from build123d import *

# Parameters (mm, degrees)
CROQUIS1_W            = 42.3
CROQUIS1_H            = 42.3
EXTRUDE_FEATURE_DEPTH = 7.6
SKETCH2_R             = 29.910616844
SKETCH2_R_2           = 27
CUT_EXTRUDE1_DEPTH    = 8.6
CROQUIS5_R            = 1.5
CORTAR_EXTRUIR2_DEPTH = 22
CROQUIS6_R            = 4.5
CORTAR_EXTRUIR3_DEPTH = 8.6
SKETCH3_R             = 5.5
CUT_EXTRUDE2_DEPTH    = 4.6
CROQUIS7_R            = 3
CORTAR_EXTRUIR4_DEPTH = 3
SKETCH1_W             = 16
SKETCH1_H             = 4.4
BOSS_EXTRUDE1_DEPTH   = 3
FILLET1_R             = 1
CHAMFER1_SIZE         = 0.5


with BuildPart() as part:
    # Croquis1 → Extrude Feature (new body)
    with BuildSketch(Plane.XY):
        Rectangle(CROQUIS1_W, CROQUIS1_H)
    extrude(amount=EXTRUDE_FEATURE_DEPTH)

    # Sketch2 → Cut-Extrude1 (cut, through all)
    with BuildSketch(Plane.XY.offset(7.6)):
        Circle(SKETCH2_R)
        Circle(SKETCH2_R_2, mode=Mode.SUBTRACT)
    extrude(amount=-CUT_EXTRUDE1_DEPTH, mode=Mode.SUBTRACT)

    # Croquis5 → Cortar-Extruir2 (cut)
    with BuildSketch(Plane(origin=(0, 0, 0), x_dir=(-1, 0, 0), z_dir=(0, 0, -1))):
        with Locations((-15.5, 15.5)):
            Circle(CROQUIS5_R)
        with Locations((15.5, 15.5)):
            Circle(CROQUIS5_R)
        with Locations((15.5, -15.5)):
            Circle(CROQUIS5_R)
        with Locations((-15.5, -15.5)):
            Circle(CROQUIS5_R)
    extrude(amount=-CORTAR_EXTRUIR2_DEPTH, mode=Mode.SUBTRACT)

    # Croquis6 → Cortar-Extruir3 (cut, through all)
    with BuildSketch(Plane(origin=(0, 0, 0), x_dir=(-1, 0, 0), z_dir=(0, 0, -1))):
        Circle(CROQUIS6_R)
    extrude(amount=-CORTAR_EXTRUIR3_DEPTH, mode=Mode.SUBTRACT)

    # Sketch3 → Cut-Extrude2 (cut)
    with BuildSketch(Plane.XY.offset(7.6)):
        Circle(SKETCH3_R)
    extrude(amount=-CUT_EXTRUDE2_DEPTH, mode=Mode.SUBTRACT)

    # Croquis7 → Cortar-Extruir4 (cut)
    with BuildSketch(Plane(origin=(0, 0, 0), x_dir=(-1, 0, 0), z_dir=(0, 0, -1))):
        with Locations((-15.5, 15.5)):
            Circle(CROQUIS7_R)
        with Locations((15.5, 15.5)):
            Circle(CROQUIS7_R)
        with Locations((15.5, -15.5)):
            Circle(CROQUIS7_R)
        with Locations((-15.5, -15.5)):
            Circle(CROQUIS7_R)
    extrude(amount=-CORTAR_EXTRUIR4_DEPTH, mode=Mode.SUBTRACT)

    # Sketch1 → Boss-Extrude1 (add)
    with BuildSketch(Plane(origin=(0, 0, 0), x_dir=(-1, 0, 0), z_dir=(0, 0, -1))):
        with Locations((0, 23.35)):
            Rectangle(SKETCH1_W, SKETCH1_H)
    extrude(amount=-BOSS_EXTRUDE1_DEPTH)

    # Fillet1
    fillet1_edges = [part.edges().sort_by_distance(p)[0] for p in [
        (-12.39162529, 21.15, 0),
        (-8, 23.35, 0),
        (0, 25.55, 0),
        (8, 23.35, 0),
        (21.15, 0, 0),
        (0, -21.15, 0),
        (-21.15, 0, 0),
        (12.39162529, 21.15, 0),
        (19.091883092, -19.091883092, 0),
        (-19.091883092, -19.091883092, 0),
        (-19.091883092, 19.091883092, 0),
        (19.091883092, 19.091883092, 0),
    ]]
    fillet(fillet1_edges, radius=FILLET1_R)

    # Chamfer1
    chamfer1_edges = [part.edges().sort_by_distance(p)[0] for p in [
        (18.5, 15.5, 0),
        (-12.5, 15.5, 0),
        (-12.5, -15.5, 0),
        (18.5, -15.5, 0),
    ]]
    chamfer(chamfer1_edges, length=CHAMFER1_SIZE)


solid = part.part
The model under review builds one solid part; all positions refer to its coordinate system, in mm. A direction names the side the tool comes from. Give positions to 0.01 mm unless a question says otherwise; leave off trailing zeros. Write each loop counter-clockwise with the first axis right and the second up, starting at its lowest first coordinate (ties: lowest second). Pieces come first, ordered by that corner, then holes.
1. Tool access review of faces 5 (the cylindrical face through (11.96, 20.849, 0.285)), 6 (the flat face through (-17, 14, 3)), 7 (the cylindrical face through (-1.19, -5.37, 5.33)): name each direction out of +Z, -Z, +X, -X, +Y, -Y from which nothing blocks a thin tool from reaching the whole face with its end or side.
2. Wall thickness on L1, parallel to Y at x = 15.5, z = 6.75; L2, parallel to X at y = 18, z = 1: over which ranges is each line inside the solid? List them lowest first.
3. Add section C-C, the plane z = 1.75. Write out the cut boundary in (x, y), plus the area to 3 significant figures.
4. For P1, Ø0.6, axis at y = 24, z = 2.5, coming from the -X side; P2, Ø3.5, axis at x = -15.5, y = -15.5, coming from the -Z side; P3, Ø1, axis at x = 1, y = 3, coming from the -Z side; P4, Ø1.5, axis at x = -10.5, z = 7, coming from the +Y side, all flat-tipped, find the tip position at first contact; note any pin that passes through.
5. Add section D-D, the plane x = -3. Write out the cut boundary in (y, z), plus the area to 3 significant figures.
6. Add section A-A, the plane x = -15.5. Write out the cut boundary in (y, z).
7. Draft analysis for pull direction Y (two halves, no side actions). For faces 1 (the cylindrical face through (17, 15.57, 5.27)), 2 (the flat face through (0, -21.15, 4)), 3 (the flat face through (0, 25.55, 2)), 4 (the cylindrical face through (-20.865, 0.235, 0.301)), state which applies: +Y half, -Y half, draft (parallel to the pull), parting line (faces both ways), or undercut.
8. Add section B-B, the plane y = 0. Write out the cut boundary in (x, z), plus the area to 3 significant figures.
Worked answers:
1. face 5: -Z, +X, +Y
1. face 6: -Z
1. face 7: +Z
2. L1: y = -21.15 to -17, -14 to 14, 17 to 21.15
2. L2: x = -20.12 to -17.16, -13.84 to 13.84, 17.16 to 20.12
3. outline: (-21.15, -16.78) arc R27 ccw to (-16.78, -21.15) - (16.78, -21.15) arc R27 ccw to (21.15, -16.78) - (21.15, 16.78) arc R27 ccw to (16.78, 21.15) - (8, 21.15) - (8, 25.55) - (-8, 25.55) - (-8, 21.15) - (-16.78, 21.15) arc R27 ccw to (-21.15, 16.78) - close; hole circle Ø6 at (-15.5, -15.5); hole circle Ø6 at (-15.5, 15.5); hole circle Ø9 at (0, 0); hole circle Ø6 at (15.5, -15.5); hole circle Ø6 at (15.5, 15.5)
3. area: 1,650 mm2
4. P1: stops at x = -8
4. P2: stops at z = 3
4. P3: passes through
4. P4: stops at y = 21.15
5. outline: (-21.15, 1) arc R1 ccw to (-20.15, 0) - (-3.35, 0) - (-3.35, 3) - (-4.61, 3) - (-4.61, 7.6) - (-21.15, 7.6) - close; (3.35, 0) - (24.55, 0) arc R1 ccw to (25.55, 1) - (25.55, 3) - (21.15, 3) - (21.15, 7.6) - (4.61, 7.6) - (4.61, 3) - (3.35, 3) - close
5. area: 272 mm2
6. outline: (-21.15, 1) arc R1 ccw to (-20.15, 0) - (-19, 0) - (-18.5, 0.5) - (-18.5, 3) - (-17, 3) - (-17, 7.6) - (-21.15, 7.6) - close; (-14, 3) - (-12.5, 3) - (-12.5, 0.5) - (-12, 0) - (12, 0) - (12.5, 0.5) - (12.5, 3) - (14, 3) - (14, 7.6) - (-14, 7.6) - close; (17, 3) - (18.5, 3) - (18.5, 0.5) - (19, 0) - (20.15, 0) arc R1 ccw to (21.15, 1) - (21.15, 7.6) - (17, 7.6) - close
7. face 1: undercut
7. face 2: -Y half
7. face 3: +Y half
7. face 4: draft
8. outline: (-21.15, 1) arc R1 ccw to (-20.15, 0) - (-4.5, 0) - (-4.5, 3) - (-5.5, 3) - (-5.5, 7.6) - (-21.15, 7.6) - close; (4.5, 0) - (20.15, 0) arc R1 ccw to (21.15, 1) - (21.15, 7.6) - (5.5, 7.6) - (5.5, 3) - (4.5, 3) - close
8. area: 243 mm2
